Could you check a few things on this model? Use its own coordinates, in mm. A direction names the side the tool comes from. Give positions to 0.01 mm unless a question says otherwise; leave off trailing zeros. Loops run counter-clockwise (first coordinate to the right, second up) from the corner with the lowest first, then second, coordinate; pieces in that order, holes last. Notation, with made-up numbers: (35, 33) -> (52, 33) arc R12 ccw to (52, 49) -> close; hole circle Ø8 at (-29, -0.75). An arc over 180 degrees is marked (long way). Put each result on its own line as item: value.
Autodesk Inventor part; units mm, degrees
ref_plane "Work Plane2" through (-2.9345, 5.0828, 0) normal (-0.866, -0.5, 0) x (0, 0, 1)
ref_plane "Work Plane3" through (0, 0, 1.5875) normal (0, 0, 1) x (1, 0, 0)
ref_plane "YZ Plane" through (0, 0, 0) normal (1, 0, 0) x (0, 1, 0)
sketch "Sketch1" plane through (0, 0, 0) normal (0, 0, 1) x (1, 0, 0)
  circle A0 centre (0, 0) radius 2.2479
  circle A1 centre (-1.3525, -2.3427) radius 0.4572
  circle A2 centre (1.3526, -2.3427) radius 0.4572
  circle A3 centre (2.7051, 0) radius 0.4572
  circle A4 centre (1.3525, 2.3427) radius 0.4572
  circle A5 centre (-1.3525, 2.3427) radius 0.4572
  circle A6 centre (-2.7051, 0) radius 0.4572
  line L0 (-1.6165, -2.7999) -> (-3.233, 0)
  line L1 (-3.233, 0) -> (-1.6165, 2.7999)
  line L2 (-1.6165, 2.7999) -> (1.6165, 2.7999)
  line L3 (1.6165, 2.7999) -> (3.233, 0)
  line L4 (3.233, 0) -> (1.6165, -2.7999)
  line L5 (1.6165, -2.7999) -> (-1.6165, -2.7999)
  line L6 (0, 0) -> (0, -5.0828)
  line L7 (-5.8691, 0) -> (-2.9345, 5.0828)
  line L8 (-2.9345, 5.0828) -> (2.9345, 5.0828)
  line L9 (2.9345, 5.0828) -> (5.8691, 0)
  line L10 (2.9345, -5.0828) -> (-2.9345, -5.0828)
  line L11 (-2.9345, -5.0828) -> (-5.8691, -5.0828)
  line L12 (-5.8691, -5.0828) -> (-5.8691, 0)
  line L13 (2.9345, -5.0828) -> (5.8691, -5.0828)
  line L14 (5.8691, -5.0828) -> (5.8691, 0)
  point P0 (0, -2.2479)
  dimension "d0" = 4.4958
  dimension "d4" = 360
extrude "Extrusion1" add sketch "Sketch1" along normal blind 3.175
sketch "Sketch2" plane through (0, 0, 3.175) normal (0, 0, 1) x (1, 0, 0)
  line L0 (2.9345, 5.0828) -> (-2.9345, 5.0828)
  circle A0 centre (-8.2426, 2.2407) radius 1.5
  circle A1 centre (-4.4104, 7.7112) radius 1.5
  circle A2 centre (-12.2306, -3.4521) radius 1.6091
  line L1 (0, -1.718) -> (0, 5.1689)
  circle A3 centre (8.2426, 2.2407) radius 1.5
  circle A4 centre (12.2306, -3.4521) radius 1.6091
  circle A5 centre (4.4104, 7.7112) radius 1.5
  line L2 (-5.8691, 0) -> (-10.6162, -6.6427)
  line L3 (-10.6162, -6.6427) -> (-15.4056, -6.6427)
  line L4 (-15.4056, -6.6427) -> (-15.4056, -0.2771)
  line L5 (-15.4056, -0.2771) -> (-6.6459, 10.2346)
  line L6 (-6.6459, 10.2346) -> (0, 10.2346)
  line L7 (5.8691, 0) -> (10.6162, -6.6427)
  line L8 (10.6162, -6.6427) -> (15.4056, -6.6427)
  line L9 (15.4056, -6.6427) -> (15.4056, -0.2771)
  line L10 (15.4056, -0.2771) -> (6.6459, 10.2346)
  line L11 (6.6459, 10.2346) -> (0, 10.2346)
  line L12 (5.8691, 0) -> (2.9345, 5.0828)
  line L13 (5.8691, 0) -> (2.9345, 5.0828)
  line L14 (2.9345, 5.0828) -> (-2.9345, 5.0828)
  line L15 (5.8691, 0) -> (2.9345, 5.0828)
  line L16 (-5.8691, 0) -> (-2.9345, 5.0828)
  line L17 (-4.4104, 7.7112) -> (-12.2306, -3.4521)
  point P0 (-2.9579, 5.0828)
  dimension "d28" = 3
  dimension "d29" = 3
  dimension "d30" = 9.144
ref_plane "Work Plane2" through (-2.9345, 5.0828, 0) normal (-0.866, -0.5, 0) x (0, 0, 1)
ref_plane "Work Plane3" through (0, 0, 1.5875) normal (0, 0, 1) x (1, 0, 0)
extrude "Extrusion4" add sketch "Sketch2" against normal blind 3.175
properties part number "WireGuideBoltHols"
1. For faces 1 (the face through (5.869, -3, 2)), 2 (the face through (-15.406, -4, 2)), 3 (the face through (0, -2.8, 2)), which set-ups out of +Z, -Z, +X, -X, +Y, -Y let a thin tool reach every point of the face, with its end or its side?
Recorded:
face 1: +Z, -Z, -Y
face 2: +Z, -Z, -X, +Y, -Y
face 3: +Z, -Z
2. I need wall thicknesses on line 1 (X direction, y = -2.25, z = 1.35); line 2 (X direction, y = 2.25, z = 0.4); line 3 (X direction, y = 7.25, z = 2.6). Which ranges of each line are inside material? Lowest first, please.
Recorded:
line 1: x = -15.41 to -13.3, -11.16 to -7.48, -5.87 to -1.93, 1.93 to 5.87, 7.48 to 11.16, 13.3 to 15.41
line 2: x = -13.3 to -9.74, -6.74 to -1.93, 1.93 to 6.74, 9.74 to 13.3
line 3: x = -9.13 to -5.84, -2.98 to 2.98, 5.84 to 9.13
3. If we section it at B-B (x = -12): List the corners of the cut face in (y, z) for me (3 decimals).
Recorded:
outline: (-6.643, 0) -> (-5.045, 0) -> (-5.045, 3.175) -> (-6.643, 3.175) -> close; (-1.86, 0) -> (3.81, 0) -> (3.81, 3.175) -> (-1.86, 3.175) -> close
4. Thinking about a two-plate mould opening in Y: for faces 4 (the face through (0, -5.083, 2)), 5 (the face through (13.717, -4.068, 1.61)), 6 (the face through (-11.087, 4.905, 1.61)), which applies, pulls with the +Y half, pulls with the -Y half, needs draft (parallel to the pull), parting line crosses it, or undercut?
Recorded:
face 4: pulls with the -Y half
face 5: undercut
face 6: pulls with the +Y half
5. I'm going to push flat-ended pins straight in: pin 1 (1.8 mm diameter, centred on x = 8.24, y = 2.24, fed in from -Z); pin 2 (1 mm diameter, centred on x = 0.5, z = 2, fed in from -Y). Where does each tip first touch, or does it pass through?
Recorded:
pin 1: passes through
pin 2: stops at y = -5.08
6. If we section it at D-D (z = 1): List the corners of the cut face in (x, y) for me.
Recorded:
outline: (-15.41, -6.64) -> (-10.62, -6.64) -> (-5.87, 0) -> (-5.87, -5.08) -> (5.87, -5.08) -> (5.87, 0) -> (10.62, -6.64) -> (15.41, -6.64) -> (15.41, -0.28) -> (6.65, 10.23) -> (-6.65, 10.23) -> (-15.41, -0.28) -> close; hole circle Ø3.22 at (-12.23, -3.45); hole circle Ø3 at (-8.24, 2.24); hole circle Ø3 at (-4.41, 7.71); hole (-3.23, 0) -> (-1.62, -2.8) -> (1.62, -2.8) -> (3.23, 0) -> (1.62, 2.8) -> (-1.62, 2.8) -> close; hole circle Ø3 at (4.41, 7.71); hole circle Ø3 at (8.24, 2.24); hole circle Ø3.22 at (12.23, -3.45)
7. If we section it at C-C (y = 6.75): List the corners of the cut face in (x, z) for me (3 decimals).
Recorded:
outline: (-9.55, 0) -> (-5.562, 0) -> (-5.562, 3.175) -> (-9.55, 3.175) -> close; (-3.259, 0) -> (3.259, 0) -> (3.259, 3.175) -> (-3.259, 3.175) -> close; (5.562, 0) -> (9.55, 0) -> (9.55, 3.175) -> (5.562, 3.175) -> close
8. If we section it at A-A (y = 1.25): List the corners of the cut face in (x, z) for me (3 decimals), then the cut area to 3 significant figures.
Recorded:
outline: (-14.133, 0) -> (-9.369, 0) -> (-9.369, 3.175) -> (-14.133, 3.175) -> close; (-7.116, 0) -> (-2.511, 0) -> (-2.511, 3.175) -> (-7.116, 3.175) -> close; (2.511, 0) -> (7.116, 0) -> (7.116, 3.175) -> (2.511, 3.175) -> close; (9.369, 0) -> (14.133, 0) -> (14.133, 3.175) -> (9.369, 3.175) -> close
area: 59.5 mm^2
